Solid Edge part; units mm, degrees
sketch "Sketch1" plane through (0, 0, 0) normal (0, 0, 1) x (1, 0, 0)
  circle A0 centre (0, 0) radius 6
extrude "Protrusion1" add sketch "Sketch1" along normal mid plane 5
hole "hole" at (0, 0, 2.5) direction (0, 0, -1) diameter 3.2 depth 30 tip angle 118 start chamfer 0.6 start chamfer angle 45 end chamfer 0.6 end chamfer angle 45
sketch "Sketch2" plane through (0, 0, 2.5) normal (0, 0, 1) x (-1, 0, 0)
  line L0 (-25, -4) -> (-4.4721, -4)
  line L1 (-4.4721, -4) -> (-4.4721, 4)
  line L2 (-4.4721, 4) -> (-25, 4)
  line L3 (-25, 4) -> (-25, -4)
  dimension "D1" = 4.4721
extrude "Protrusion2" add sketch "Sketch2" against normal up to vertex (5 mm away)
sketch "Sketch3" plane through (12, 0, 2.5) normal (0, 0, 1) x (1, 0, 0)
  line L0 (13, 4) -> (5, 4)
  line L1 (5, 4) -> (5, -4)
  line L2 (5, -4) -> (13, -4)
  line L3 (13, -4) -> (13, 4)
  dimension "D1" = 13
extrude "ExtrudedProtrusion_3" add sketch "Sketch3" along normal blind 5.1
properties material "Polyethylene, low density"
Geometry check sheet. Reference: the model listing, model coordinates, mm. A direction names the side the tool comes from. Round coordinates to 2 decimals unless told otherwise and drop trailing zeros. Order: outer loops, then holes, each group sorted by start corner. A loop starts at its lowest first (then second) coordinate and runs counter-clockwise, first axis right, second up. Notation, with made-up numbers: (88.5, 88) -> (93.5, 88) arc R23 cw to (93.5, 99) -> close; hole circle Ø6 at (80.5, 14). An arc over 180 degrees is marked (long way). Return JSON: item names as keys, results as strings. Group by question number.
Q1. Gauge pin test, flat ends, axial feed: pin 1 (1.5 mm diameter, centred on y = -1.5, z = 6, fed in from -X); pin 2 (5 mm diameter, centred on x = 9, z = 4.5, fed in from +Y); pin 3 (3 mm diameter, centred on x = 17, z = 0.5, fed in from -Y). Record the tip position at first contact, or that the pin passes through.
Q2. Section check A-A, the plane x = 0. Record the boundary of the cut face in (y, z).
Q3. Tool access check on faces 1 (the cylindrical face through (-6, 0, 0)), 2 (the flat face through (21, 0, 7.6)), 3 (the flat face through (17, 4, 1)), 4 (the flat face through (17, -4, 1)), 5 (the flat face through (5, 0, 2.5)). Record the directions out of +Z, -Z, +X, -X, +Y, -Y that give a thin tool (end or side, any length) a straight path to the whole face; none if there is none.
Q4. Material ranges on probe 1 along X at (y, z) = (0, 0.4); probe 2 along Y at (x, z) = (0, -0.85); probe 3 along Z at (x, y) = (3, 3), recorded low to high. Write a range as from..to.
Q5. Section check B-B, the plane y = 0. Record the boundary of the cut face in (x, z).
Q6. Section check C-C, the plane z = -1.25. Record the boundary of the cut face in (x, y), plus the area to 3 significant figures.
Q7. Section check D-D, the plane x = 5.5. Record the boundary of the cut face in (y, z), plus the area to 3 significant figures.
Q8. Release check for a two-part mould opening along X. For faces 6 (the flat face through (25, 0, 3)), 7 (the flat face through (9, 0, -2.5)), 8 (the cylindrical face through (0.97, 1.27, -0.03)) record: released by +X, released by -X, zero draft, split by the parting line, or undercut.
Numbers:
{
 "1": {"pin 1": "x = 17", "pin 2": "y = 4", "pin 3": "y = -4"},
 "2": {"outline": "(-6, -2.5) -> (-2.2, -2.5) -> (-1.6, -1.9) -> (-1.6, 1.9) -> (-2.2, 2.5) -> (-6, 2.5) -> close; (1.6, -1.9) -> (2.2, -2.5) -> (6, -2.5) -> (6, 2.5) -> (2.2, 2.5) -> (1.6, 1.9) -> close"},
 "3": {"face 1": "+Z, -Z", "face 2": "+Z, +X, -X, +Y, -Y", "face 3": "+Z, -Z, +X, +Y", "face 4": "+Z, -Z, +X, -Y", "face 5": "+Z, -X, +Y, -Y"},
 "4": {"probe 1": "-6..-1.6, 1.6..25", "probe 2": "-6..-1.6, 1.6..6", "probe 3": "-2.5..2.5"},
 "5": {"outline": "(-6, -2.5) -> (-2.2, -2.5) -> (-1.6, -1.9) -> (-1.6, 1.9) -> (-2.2, 2.5) -> (-6, 2.5) -> close; (1.6, -1.9) -> (2.2, -2.5) -> (25, -2.5) -> (25, 7.6) -> (17, 7.6) -> (17, 2.5) -> (2.2, 2.5) -> (1.6, 1.9) -> close"},
 "6": {"outline": "(4.47, -4) -> (25, -4) -> (25, 4) -> (4.47, 4) arc R6 ccw (long way) to start; hole circle Ø3.2 at (0, 0)", "area": "261 mm^2"},
 "7": {"outline": "(-4, -2.5) -> (4, -2.5) -> (4, 2.5) -> (-4, 2.5) -> close", "area": "40.0 mm^2"},
 "8": {"face 6": "released by +X", "face 7": "zero draft", "face 8": "undercut"}
}
